Model file for the job. Use its own axes, mm. Give positions to 0.01 mm unless a question says otherwise; leave off trailing zeros. Write each loop counter-clockwise with the first axis right and the second up, starting at its lowest first coordinate (ties: lowest second). Pieces come first, ordered by that corner, then holes. Notation, with made-up numbers: (38, -2) - (58, -2) arc R22 ccw to (58, 37) - close; hole circle Ø6 at (67.25, 73.25). An arc over 180 degrees is marked (long way). One line per item, written item: value. Start each with the question number.
(1) Cut at A-A, the plane x = -35.4. List the corners of the cut face in (y, z), and give its area (3 significant figures).
(2) Probe L1, parallel to X at y = -3.6, z = 62.5; L2, parallel to X at y = -3.4, z = 70; L3, parallel to Y at x = -34, z = 26. List the from-to ranges inside material, lowest first.
(3) Cut at D-D, the plane y = -1.5. List the corners of the cut face in (x, z), and give its area (3 significant figures).
(4) Cut at C-C, the plane x = -20. List the corners of the cut face in (y, z), and give its area (3 significant figures).
(5) Drop a flat-ended pin along its axis: P1, Ø10, axis at x = -23, z = 31.5, coming from the +Y side. Give the stop position or say it passes through.
(6) Cut at B-B, the plane z = 4. List the corners of the cut face in (x, y).
from build123d import *

# Parameters (mm, degrees)
SKETCH1_W           = 92.8
SKETCH1_H           = 124.8
BOSS_EXTRUDE1_DEPTH = 2
CUT_EXTRUDE1_DEPTH  = 92.082431134


with BuildPart() as part:
    # Sketch1 → Boss-Extrude1 (new body)
    with BuildSketch(Plane(origin=(0, -2.3, 0), x_dir=(-1, 0, 0), z_dir=(0, -1, 0))):
        with Locations((-1, -15.351201027)):
            Rectangle(SKETCH1_W, SKETCH1_H)
    extrude(amount=BOSS_EXTRUDE1_DEPTH)

    # Sketch3 → Revolve2 (revolve)
    with BuildSketch(Plane.ZY.offset(-1), mode=Mode.PRIVATE) as revolve2_sk:
        with BuildLine():
            Line((8.11798754, -2.3), (10.61798754, -2.3))
            Line((10.61798754, -2.3), (10.61798754, -0.3))
            ThreePointArc((10.61798754, -0.3), (9.017206481, -0.861523676), (8.11798754, -2.3))
        make_face()
    revolve(revolve2_sk.sketch.rotate(Axis((1, -0.3, 10.61798754), (0, -1, 0)), 180), axis=Axis((1, -0.3, 10.61798754), (0, -1, 0)))

    # Sketch5 → Revolve3 (revolve)
    with BuildSketch(Plane.ZY.offset(-1)):
        with BuildLine():
            Line((20.10120103, -2.3), (20.10120103, -0.3))
            ThreePointArc((20.10120103, -0.3), (18.500419971, -0.861523676), (17.60120103, -2.3))
            Line((17.60120103, -2.3), (20.10120103, -2.3))
        make_face()
    revolve(axis=Axis((1, -2.3, 20.10120103), (0, 1, 0)))

    # Sketch6 → Cut-Extrude1 (cut, through all)
    with BuildSketch(Plane(origin=(0, -2.3, 0), x_dir=(1, 0, 0), z_dir=(0, 1, 0))):
        with BuildLine():
            Line((-30.4, 37.048798973), (-30.4, 27.565585483))
            ThreePointArc((-30.4, 27.565585483), (-35.4, 22.565585483), (-40.4, 27.565585483))
            Line((-40.4, 27.565585483), (-40.4, 37.048798973))
            ThreePointArc((-40.4, 37.048798973), (-35.4, 42.048798973), (-30.4, 37.048798973))
        make_face()
        with BuildLine():
            Line((-30.4, -58.267987537), (-30.4, -67.751201027))
            ThreePointArc((-30.4, -67.751201027), (-35.4, -72.751201027), (-40.4, -67.751201027))
            Line((-40.4, -67.751201027), (-40.4, -58.267987537))
            ThreePointArc((-40.4, -58.267987537), (-35.4, -53.267987537), (-30.4, -58.267987537))
        make_face()
    cut_extrude1 = extrude(amount=-CUT_EXTRUDE1_DEPTH, mode=Mode.SUBTRACT)

    # Mirror1: Cut-Extrude1 across plane
    add(cut_extrude1.mirror(Plane.ZY.offset(-1)), mode=Mode.SUBTRACT)


solid = part.part
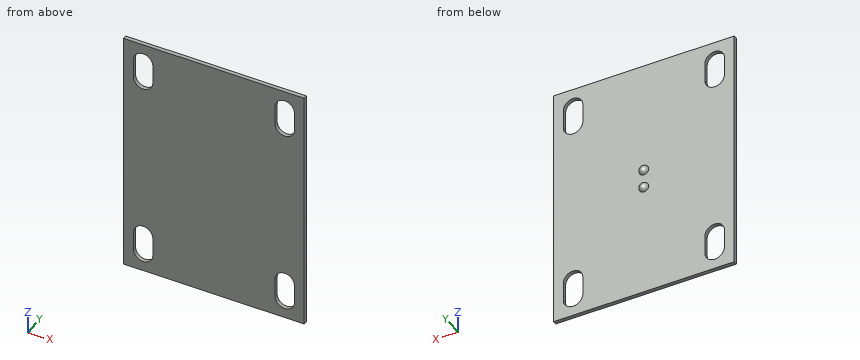
Answers follow:
1. outline: (-4.3, -47.05) - (-2.3, -47.05) - (-2.3, -42.05) - (-4.3, -42.05) - close; (-4.3, -22.57) - (-2.3, -22.57) - (-2.3, 53.27) - (-4.3, 53.27) - close; (-4.3, 72.75) - (-2.3, 72.75) - (-2.3, 77.75) - (-4.3, 77.75) - close
1. area: 172 mm²
2. L1: x = -45.4 to -40.4, -30.4 to 32.4, 42.4 to 47.4
2. L2: x = -45.4 to -39.87, -30.93 to 32.93, 41.87 to 47.4
2. L3: y = -4.3 to -2.3
3. outline: circle Ø4.34 at (1, 10.62); circle Ø4.34 at (1, 20.1)
3. area: 29.6 mm²
4. outline: (-4.3, -47.05) - (-2.3, -47.05) - (-2.3, 77.75) - (-4.3, 77.75) - close
4. area: 250 mm²
5. P1: stops at y = -2.3
6. outline: (-45.4, -4.3) - (47.4, -4.3) - (47.4, -2.3) - (-45.4, -2.3) - close
